Geometry check sheet. Reference: drawing and pictorial views, mm from the part's lowest x, y, z. A direction names the side the tool comes from. Coordinates: 2 decimals unless noted, no trailing zeros. Loops run counter-clockwise (first coordinate to the right, second up) from the corner with the lowest first, then second, coordinate; pieces in that order, holes last. Notation, with made-up numbers: (32.5, 19.5) - (75.5, 19.5) arc R9 cw to (75.5, 28.5) - close; hole circle Ø1 at (35, 48). An arc over 180 degrees is marked (long way). One line per item, written item: value.
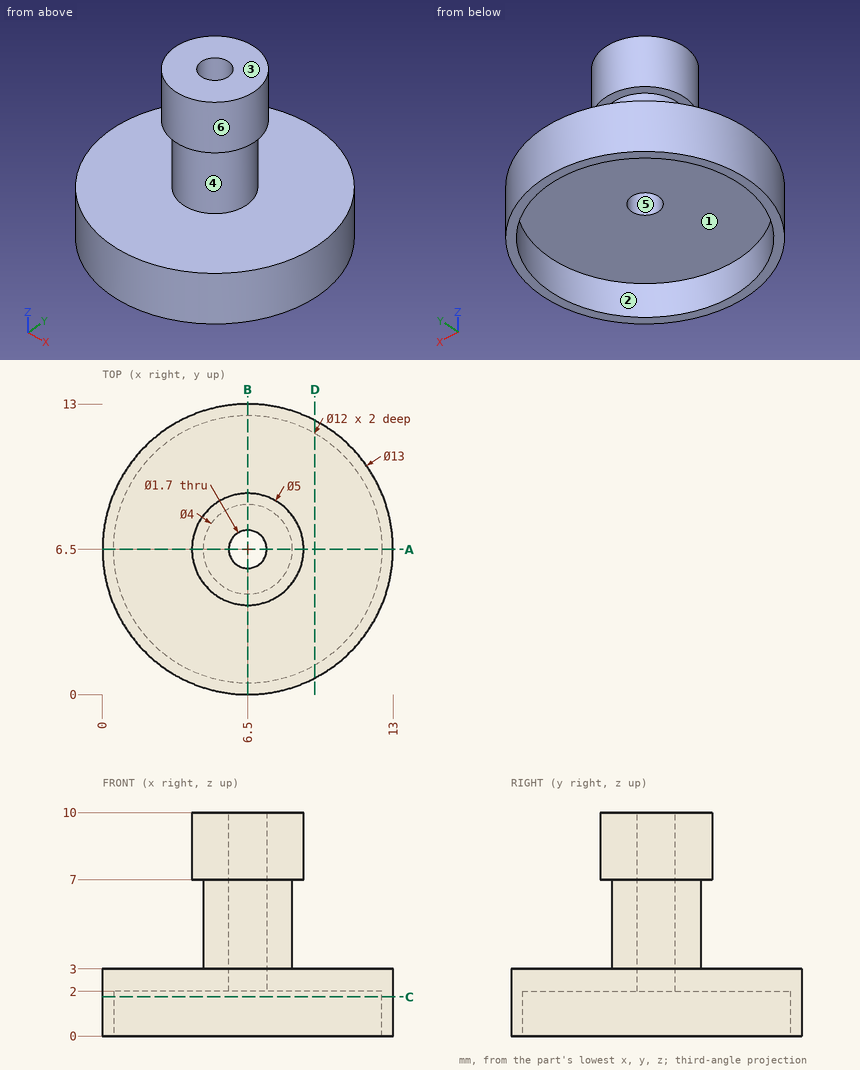
(1) Cross-section at D-D on x = 9.5. Record the cut outline in (y, z).
Reply:
outline: (0.73, 0) - (1.3, 0) - (1.3, 2) - (11.7, 2) - (11.7, 0) - (12.27, 0) - (12.27, 3) - (0.73, 3) - close
(2) Release check for a two-part mould opening along Z. For the marked faces 1, 2, 3 and 4 record: pulls with the +Z half, pulls with the -Z half, needs draft (parallel to the pull), parting line crosses it, or undercut.
Reply:
face 1: pulls with the -Z half
face 2: needs draft
face 3: pulls with the +Z half
face 4: undercut
(3) Cross-section at A-A on y = 6.5. Record the cut outline in (x, z), and give its area (3 significant figures).
Reply:
outline: (0, 0) - (0.5, 0) - (0.5, 2) - (5.65, 2) - (5.65, 10) - (4, 10) - (4, 7) - (4.5, 7) - (4.5, 3) - (0, 3) - close; (7.35, 2) - (12.5, 2) - (12.5, 0) - (13, 0) - (13, 3) - (8.5, 3) - (8.5, 7) - (9, 7) - (9, 10) - (7.35, 10) - close
area: 32.4 mm2
(4) Access from +Z, -Z, +X, -X, +Y, -Y to the whole of each face (thin tool, end or side, straight path). Record for the marked faces 5 and 6.
Reply:
face 5: +Z, -Z
face 6: +Z
(5) Material ranges on probe 1 along Y at (x, z) = (6.5, 6); probe 2 along Y at (x, z) = (6.5, 0.65); probe 3 along Z at (x, y) = (10, 9), recorded low to high. Write a range as from..to.
Reply:
probe 1: 4.5..5.65, 7.35..8.5
probe 2: 0..0.5, 12.5..13
probe 3: 2..3
(6) Go/stop test with flat-tipped pins: pin 1 Ø3 at (x, y) = (2, 10) entering from +Z; pin 2 Ø2 at (x, y) = (6.5, 6.5) entering from -Z; pin 3 Ø1 at (y, z) = (8, 7.5) entering from -X. Record where each tip stops, or that it passes through.
Reply:
pin 1: z = 3
pin 2: z = 2
pin 3: x = 4.21
(7) Cross-section at C-C on z = 1.75. Record the cut outline in (x, y).
Reply:
outline: circle Ø13 at (6.5, 6.5); hole circle Ø12 at (6.5, 6.5)
